Source: CAD feature listing. Evaluate the final solid. Frame: model axes, mm. Face numbers are marked on the shaded views. A direction names the side the tool comes from. Coordinates: 2 decimals unless noted, no trailing zeros. Loops run counter-clockwise (first coordinate to the right, second up) from the corner with the lowest first, then second, coordinate; pieces in that order, holes last.
Item 1: Reachability of the marked faces 4 and 5 from +Z, -Z, +X, -X, +Y, -Y: full face, straight path, thin tool, end or side. Return the list, or none.
Item 2: Line query: probe 1 along Z at (x, y) = (3.8, 0) (3 decimals); probe 2 along Z at (x, y) = (2.55, 0); probe 3 along Z at (x, y) = (1.1, -0.75). Output: solid intervals per line, ascending.
Item 3: Pin query (flat end, axial travel): pin 1 Ø1.5 at (x, y) = (2, -1.5) entering from -Z; pin 2 Ø4 at (y, z) = (0, 0) entering from -X. Return the tip coordinate at first contact, or that it passes through.
Item 4: Section query C-C, the plane x = 1.4. Return the cut outline in (y, z), then the cut area to 3 significant figures.
Item 5: Pull-direction query (Z, two-part tool) for the marked faces 1, 2 and 3; classes: +Z half, -Z half, draft (parallel to the pull), parting line (faces both ways), or undercut.
Autodesk Inventor part; units mm, degrees
ref_plane "to_housing_XY" through (0, 0, 0) normal (1, 0, 0) x (0, 0, -1)
ref_plane "to_housing_YZ" through (0, 0, 0) normal (0, 0, -1) x (0, 1, 0)
ref_plane "to_housing_ZX" through (0, 0, 0) normal (0, 1, 0) x (1, 0, 0)
sketch "Sketch_1" plane through (0, 0, 0) normal (0, 0, 1) x (1, 0, 0)
  line L0 (3.85, 0) -> (0.15, 0)
  arc A0 (0, 2.65) -> (0.15, 2.5) centre (0.15, 2.65) ccw
  line L1 (0.15, 2.5) -> (3.85, 2.5)
  arc A1 (3.85, 2.5) -> (4, 2.65) centre (3.85, 2.65) ccw
  line L2 (4, 2.65) -> (4, 3.69)
  line L3 (4, 3.69) -> (3.7344, 3.69)
  line L4 (3.7344, 3.69) -> (3.7344, 4.595)
  line L5 (3.7344, 4.595) -> (4, 4.595)
  line L6 (4, 4.595) -> (4, 5.35)
  arc A2 (4, 5.35) -> (3.85, 5.5) centre (3.85, 5.35) ccw
  line L7 (3.85, 5.5) -> (0.15, 5.5)
  arc A3 (0.15, 5.5) -> (0, 5.35) centre (0.15, 5.35) ccw
  line L8 (0, 5.35) -> (0, 4.595)
  line L9 (0, 4.595) -> (0.2656, 4.595)
  line L10 (0.2656, 4.595) -> (0.2656, 3.69)
  line L11 (0.2656, 3.69) -> (0, 3.69)
  line L12 (0, 3.69) -> (0, 2.65)
revolve "Revolution1" add sketch "Sketch_1" angle 360 about axis through (3.85, 0, 0) along (1, 0, 0)
ref_plane "to_housing_XY" through (0, 0, 0) normal (1, 0, 0) x (0, 0, -1)
ref_plane "to_housing_YZ" through (0, 0, 0) normal (0, 0, -1) x (0, 1, 0)
ref_plane "to_housing_ZX" through (0, 0, 0) normal (0, 1, 0) x (1, 0, 0)
ref_plane "to_housing_center_XY" through (2, 0, 0) normal (1, 0, 0) x (0, 0, -1)
ref_plane "to_housing_center_YZ" through (2, 0, 0) normal (0, 0, -1) x (0, 1, 0)
ref_plane "to_housing_center_ZX" through (2, 0, 0) normal (0, 1, 0) x (1, 0, 0)
properties part number "BR115ZZ"
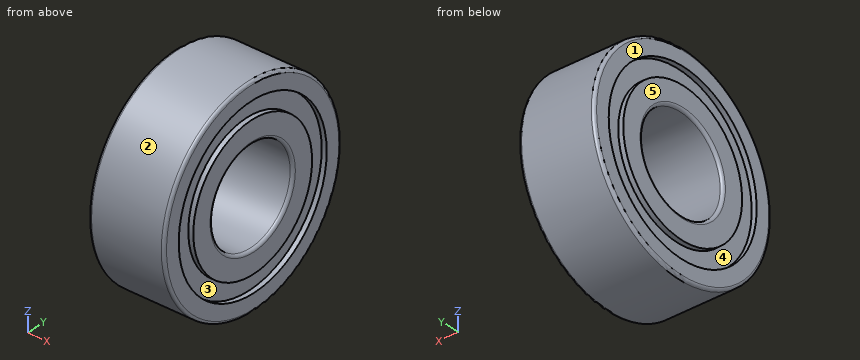
Verdict:
1. face 4: -X
1. face 5: +Z, -Z, -X, +Y, -Y
2. probe 1: z = -5.5 to -4.595, -3.69 to -2.5, 2.5 to 3.69, 4.595 to 5.5
2. probe 2: z = -5.5 to -2.5, 2.5 to 5.5
2. probe 3: z = -5.45 to -2.38, 2.38 to 5.45
3. pin 1: stops at z = -5.45
3. pin 2: passes through
4. outline: circle Ø11 at (0, 0); hole circle Ø5 at (0, 0)
4. area: 75.4 mm2
5. face 1: draft
5. face 2: parting line
5. face 3: undercut
